Verification items for this drawing (mm, ordinates from the low corner). Coordinates: 2 decimals unless noted, no trailing zeros. Loops run counter-clockwise (first coordinate to the right, second up) from the corner with the lowest first, then second, coordinate; pieces in that order, holes last.
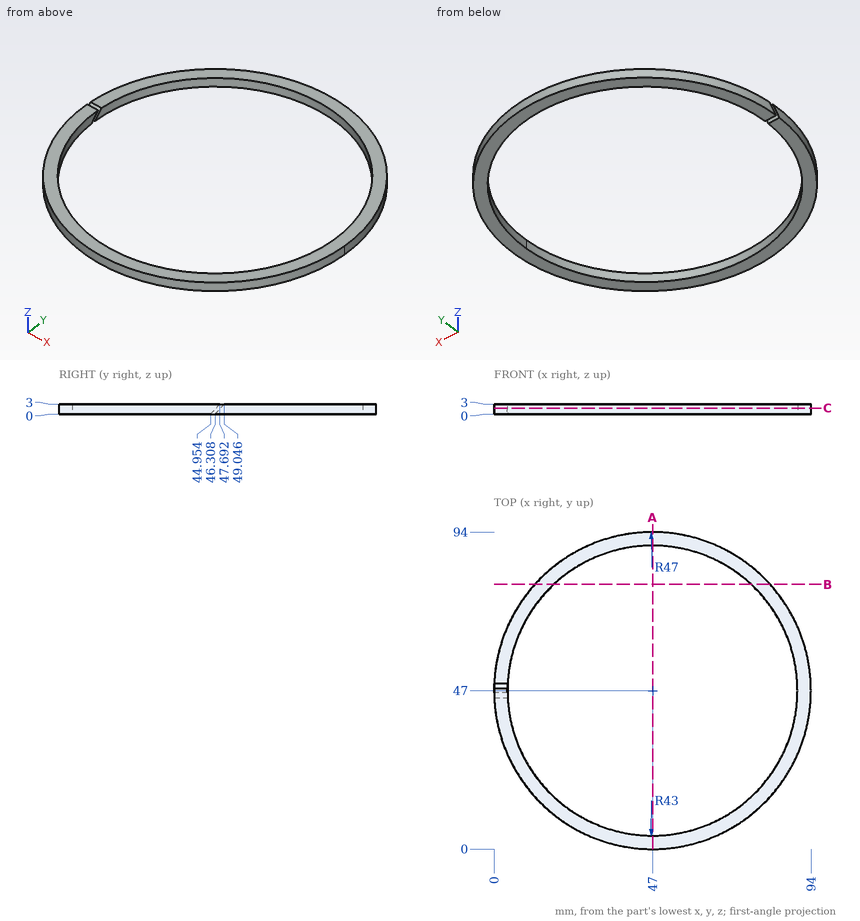
(1) Section check C-C, the plane z = 1.8. Enter the section's corners in (x, y), plus the area to 3 significant figures.
(2) Section check A-A, the plane x = 47. Enter the section's corners in (y, z).
(3) Section check B-B, the plane y = 78.5. Enter the section's corners in (x, z).
(4) Scan lines: line 1 along Y through (x, z) = (45.5, 1.3); line 2 along X through (y, z) = (11, 1.2) (1 decimal); line 3 along Y through (x, z) = (59, 2.7). Record each from-to range of solid material in increasing order.
Determined:
1. outline: (0, 46.6) arc R47 ccw (long way) to (0.01, 47.95) - (4.01, 47.95) arc R43 cw (long way) to (4, 46.6) - close
1. area: 1,130 mm2
2. outline: (0, 0) - (4, 0) - (4, 3) - (0, 3) - close; (90, 0) - (94, 0) - (94, 3) - (90, 3) - close
3. outline: (12.12, 0) - (17.73, 0) - (17.73, 3) - (12.12, 3) - close; (76.27, 0) - (81.88, 0) - (81.88, 3) - (76.27, 3) - close
4. line 1: y = 0.02 to 4.03, 89.97 to 93.98
4. line 2: x = 16.8 to 23.5, 70.5 to 77.2
4. line 3: y = 1.56 to 5.71, 88.29 to 92.44
